Autodesk Inventor part; units mm, degrees
ref_plane "YZ Plane" through (0, 0, 0) normal (1, 0, 0) x (0, 1, 0)
ref_plane "XZ Plane" through (0, 0, 0) normal (0, 1, 0) x (-1, 0, 0)
ref_plane "XY Plane" through (0, 0, 0) normal (0, 0, 1) x (1, 0, 0)
sketch "Sketch1" plane through (0, 0, 0) normal (0, 0, 1) x (1, 0, 0)
  line L0 (3, 1.7321) -> (3, -1.7321)
  line L1 (3, 1.7321) -> (0, 3.4641)
  line L2 (-3, 1.7321) -> (0, 3.4641)
  line L3 (0, -3.4641) -> (3, -1.7321)
  line L4 (-3, 1.7321) -> (-3, -1.7321)
  line L5 (-3, -1.7321) -> (0, -3.4641)
  point P0 (0, 0)
  point P1 (0, 0)
  point P2 (0, 0)
  point P3 (0, 0)
  point P4 (0, 0)
  point P5 (0, 0)
  dimension "d0" = 120
  dimension "d1" = 120
  dimension "d2" = 120
  dimension "d3" = 120
  dimension "d4" = 120
  dimension "d5" = 120
  dimension "d6" = 6
  dimension "d7" = 3
  dimension "d18" = 0
  dimension "d19" = 0
  dimension "d20" = 0
extrude "Extrusion1" add sketch "Sketch1" along normal blind 3
sketch "Sketch2" plane through (0, 0, 3) normal (0, 0, 1) x (1, 0, 0)
  circle A0 centre (0, 0) radius 1.5
  dimension "d10" = 3
extrude "Extrusion2" add sketch "Sketch2" along normal blind 6
thread "Thread2"
properties part number "m3 bolt" material "Steel, Mild"
Here's how the part is built. I have some questions about the finished solid (model axes, mm). A direction names the side the tool comes from. Coordinates: 2 decimals unless noted, no trailing zeros. Loops run counter-clockwise (first coordinate to the right, second up) from the corner with the lowest first, then second, coordinate; pieces in that order, holes last. Notation, with made-up numbers: (65, -18) -> (87, -18) arc R16 cw to (87, -11) -> close; hole circle Ø5 at (36, -2.75). An arc over 180 degrees is marked (long way). Use one line per item in the form item = value. Start each with the question number.
(1) On a 3-axis mill with a long thin cutter (end or side, diameter ignored), from which of +Z, -Z, +X, -X, +Y, -Y can I reach the whole of each face in a straight line? I mean faces 1 (the face through (-0.7, -1.5, 3)), 2 (the face through (0, 0, 9)). Say none if no direction works.
(2) Will these pins go through, and if not, where does the flat tip stop? pin 1 (2 mm diameter, centred on x = -2, y = -2.5, fed in from +Z); pin 2 (2 mm diameter, centred on y = -1.5, z = 6, fed in from -X); pin 3 (1.5 mm diameter, centred on x = 1.5, z = 4, fed in from +Y).
(3) If we section it at D-D (z = 7): Please give me the cut outline in (x, y), then the cut area to 3 significant figures.
(4) If we section it at A-A (z = 2): Please give me the cut outline in (x, y), then the cut area to 3 significant figures.
(5) Please list where these lines run through material, in increasing order: line 1 along Z through (x, y) = (-1.4, 1); line 2 along Y through (x, z) = (-0.5, 4.5); line 3 along X through (y, z) = (1, 3.5).
(6) If we section it at C-C (x = -0.95): Please give me the cut outline in (y, z), then the cut area to 3 significant figures.
(7) If we section it at B-B (y = 0): Please give me the cut outline in (x, z), then the cut area to 3 significant figures.
Verdict:
q1.face_1 = +Z
q1.face_2 = +Z, +X, -X, +Y, -Y
q2.pin_1 = 3
q2.pin_2 = -1.41
q2.pin_3 = 1.3
q3.outline = circle Ø3 at (0, 0)
q3.area = 7.07 mm²
q4.outline = (-3, -1.73) -> (0, -3.46) -> (3, -1.73) -> (3, 1.73) -> (0, 3.46) -> (-3, 1.73) -> close
q4.area = 31.2 mm²
q5.line_1 = 0 to 3
q5.line_2 = -1.41 to 1.41
q5.line_3 = -1.12 to 1.12
q6.outline = (-2.92, 0) -> (2.92, 0) -> (2.92, 3) -> (1.16, 3) -> (1.16, 9) -> (-1.16, 9) -> (-1.16, 3) -> (-2.92, 3) -> close
q6.area = 31.4 mm²
q7.outline = (-3, 0) -> (3, 0) -> (3, 3) -> (1.5, 3) -> (1.5, 9) -> (-1.5, 9) -> (-1.5, 3) -> (-3, 3) -> close
q7.area = 36.0 mm²
